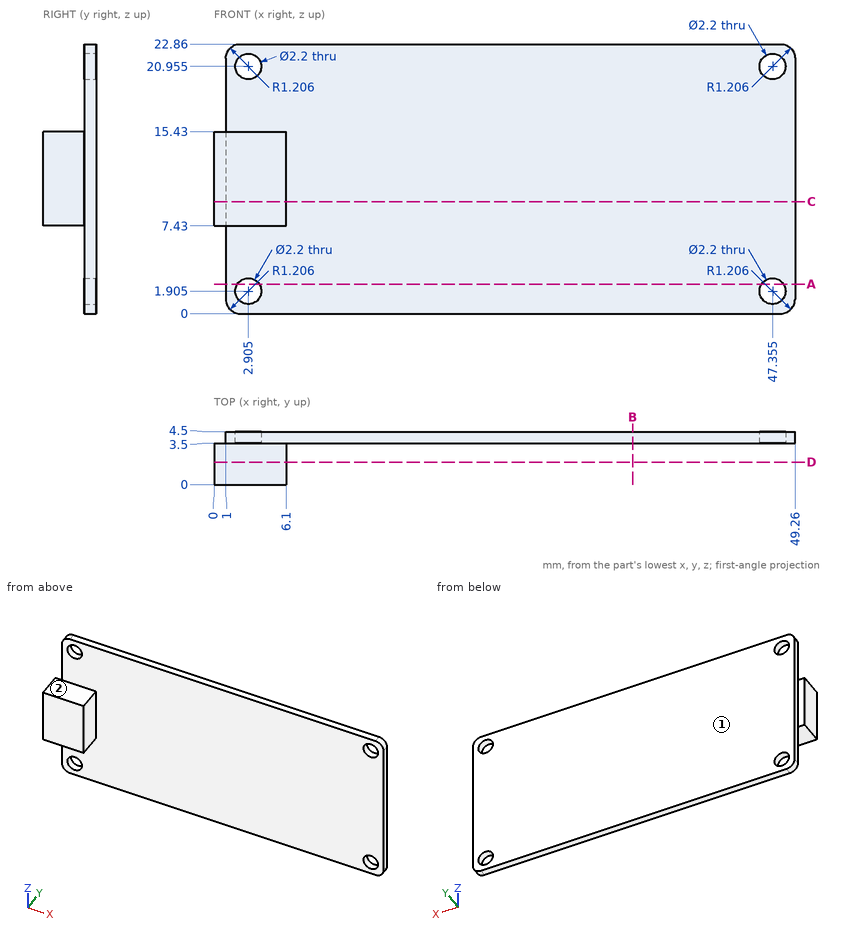
Answer from the drawing. Dimensions are ordinates in mm from the lowest x, y and z of the part. A direction names the side the tool comes from. Give positions to 0.01 mm unless a question says otherwise; leave off trailing zeros. Loops run counter-clockwise (first coordinate to the right, second up) from the corner with the lowest first, then second, coordinate; pieces in that order, holes last. Notation, with made-up numbers: (-5.5, 3.25) - (26.5, 3.25) arc R14 cw to (26.5, 18.25) - close; hole circle Ø9 at (13, 33). An arc over 180 degrees is marked (long way). Answer as a JSON object with one key per item and string values.
1. A cutting plane is placed at C-C (z = 9.5). Write down the section's boundary in (x, y).
Determined:
{"outline": "(0, 0) - (6.1, 0) - (6.1, 3.5) - (49.26, 3.5) - (49.26, 4.5) - (1, 4.5) - (1, 3.5) - (0, 3.5) - close"}
2. A cutting plane is placed at A-A (z = 2.5). Write down the section's boundary in (x, y).
Determined:
{"outline": "(1, 3.5) - (1.98, 3.5) - (1.98, 4.5) - (1, 4.5) - close; (3.83, 3.5) - (46.43, 3.5) - (46.43, 4.5) - (3.83, 4.5) - close; (48.28, 3.5) - (49.26, 3.5) - (49.26, 4.5) - (48.28, 4.5) - close"}
3. For the marked faces 1 and 2, determine the directions among +Z, -Z, +X, -X, +Y, -Y from which every point of the face is accessible in a straight line to the end or side of a thin tool.
Determined:
{"face 1": "+Z, -Z, +X, -X, +Y", "face 2": "+Z, +X, -X, -Y"}
4. Find the intervals of material crossed by L1, parallel to X at y = 4.3, z = 1.5; L2, parallel to Z at x = 3.5, y = 3.75; L3, parallel to X at y = 0.9, z = 14.75, in increasing order. Write a range as [from, to].
Determined:
{"L1": "[1, 1.88], [3.93, 46.33], [48.38, 49.26]", "L2": "[0, 0.98], [2.83, 20.03], [21.88, 22.86]", "L3": "[0, 6.1]"}
5. Flat-ended cylindrical pins translate along their axes: pin 1 Ø1.5 at (y, z) = (3.5, 19.5) entering from -X; pin 2 Ø0.5 at (x, z) = (0.5, 13) entering from +Y; pin 3 Ø2 at (x, z) = (47.355, 20.955) entering from -Y; pin 4 Ø1 at (y, z) = (1.5, 9.5) entering from +X. Find the tip coordinate at first contact, or state that the pin passes through.
Determined:
{"pin 1": "x = 1", "pin 2": "y = 3.5", "pin 3": "through", "pin 4": "x = 6.1"}
6. A cutting plane is placed at B-B (x = 35.5). Write down the section's boundary in (y, z).
Determined:
{"outline": "(3.5, 0) - (4.5, 0) - (4.5, 22.86) - (3.5, 22.86) - close"}
7. A cutting plane is placed at D-D (y = 1.9). Write down the section's boundary in (x, z).
Determined:
{"outline": "(0, 7.43) - (6.1, 7.43) - (6.1, 15.43) - (0, 15.43) - close"}
